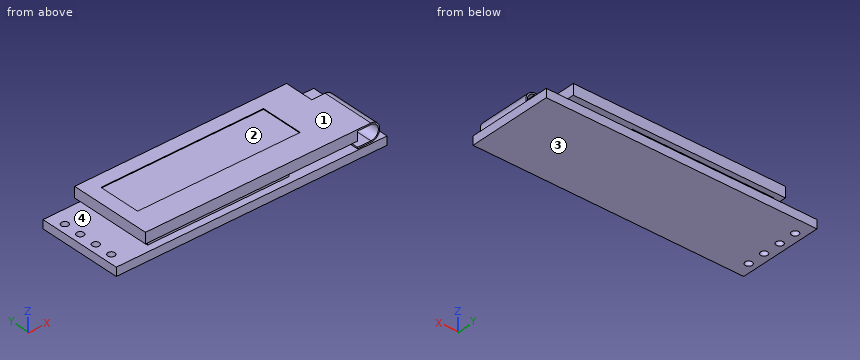
```python
from build123d import *

# Parameters (mm, degrees)
SKETCH_W     = 38.3
SKETCH_H     = 12
SKETCH_R     = 0.5
PAD_DEPTH    = 1.2
SKETCH001_W  = 20
SKETCH001_H  = 10
PAD001_DEPTH = 1
SKETCH002_W  = 30
SKETCH002_H  = 11.6
PAD002_DEPTH = 1.5
PAD003_DEPTH = 7.5
SKETCH004_W  = 23
SKETCH004_H  = 6
POCKET_DEPTH = 0.1


with BuildPart() as part:
    # Sketch → Pad (new body)
    with BuildSketch(Plane.XY):
        with Locations((17.95, 3.8)):
            Rectangle(SKETCH_W, SKETCH_H)
        Circle(SKETCH_R, mode=Mode.SUBTRACT)
        with Locations((0, 2.54)):
            Circle(SKETCH_R, mode=Mode.SUBTRACT)
        with Locations((0, 5.08)):
            Circle(SKETCH_R, mode=Mode.SUBTRACT)
        with Locations((0, 7.62)):
            Circle(SKETCH_R, mode=Mode.SUBTRACT)
    extrude(amount=PAD_DEPTH)

    # Sketch001 (on Face10 of Pad) → Pad001 (join)
    with BuildSketch(Plane.XY.offset(1.2)):
        with Locations((14.1, 3.8)):
            Rectangle(SKETCH001_W, SKETCH001_H)
    extrude(amount=PAD001_DEPTH)

    # Sketch002 (on Face15 of Pad001) → Pad002 (join)
    with BuildSketch(Plane.XY.offset(2.2)):
        with Locations((18.1, 3.8)):
            Rectangle(SKETCH002_W, SKETCH002_H)
    extrude(amount=PAD002_DEPTH)

    # Sketch003 (on Face6 of Pad002) → Pad003 (join)
    with BuildSketch(Plane.XZ.offset(2)):
        with BuildLine():
            ThreePointArc((35, 1.2), (36.25, 2.45), (35, 3.7))
            Line((33.1, 3.7), (35, 3.7))
            Line((33.1, 3.7), (33.1, 3.5))
            Line((33.1, 3.5), (35, 3.5))
            ThreePointArc((35, 1.4), (36.05, 2.45), (35, 3.5))
            Line((33.1, 1.4), (35, 1.4))
            Line((33.1, 1.4), (33.1, 1.2))
            Line((33.1, 1.2), (35, 1.2))
        make_face()
    extrude(amount=-PAD003_DEPTH)

    # Sketch004 (on Face5 of Pad003) → Pocket (cut)
    with BuildSketch(Plane.XY.offset(3.7)):
        with Locations((16.6, 4.6)):
            Rectangle(SKETCH004_W, SKETCH004_H)
    extrude(amount=-POCKET_DEPTH, mode=Mode.SUBTRACT)


solid = part.part
```
Check sheet for the modelled part. Datum: model origin and axes. Units: mm. Face numbers are marked on the shaded views. A direction names the side the tool comes from. Round coordinates to 2 decimals unless told otherwise and drop trailing zeros. Order: outer loops, then holes, each group sorted by start corner. A loop starts at its lowest first (then second) coordinate and runs counter-clockwise, first axis right, second up. Notation, with made-up numbers: (34, -0.75) - (66, -0.75) arc R24 cw to (66, 32.25) - close; hole circle Ø1 at (71, 85.25). An arc over 180 degrees is marked (long way). Write item = value, one per line.
Q1. Tool access check on the marked faces 3 and 4. Record the directions out of +Z, -Z, +X, -X, +Y, -Y that give a thin tool (end or side, any length) a straight path to the whole face; none if there is none.
Computed:
face_3 = -Z, +X, -X, +Y, -Y
face_4 = none
Q2. Section check A-A (y = 0). Record the boundary of the cut face in (x, z), and give its area (3 significant figures).
Computed:
outline = (-1.2, 0) - (-0.5, 0) - (-0.5, 1.2) - (-1.2, 1.2) - close; (0.5, 0) - (37.1, 0) - (37.1, 1.2) - (35, 1.2) arc R1.25 ccw to (35, 3.7) - (3.1, 3.7) - (3.1, 2.2) - (4.1, 2.2) - (4.1, 1.2) - (0.5, 1.2) - close; hole (24.1, 1.2) - (33.1, 1.2) - (33.1, 1.4) - (35, 1.4) arc R1.05 ccw to (35, 3.5) - (33.1, 3.5) - (33.1, 2.2) - (24.1, 2.2) - close
area = 111 mm^2
Q3. Section check B-B (x = 17). Record the boundary of the cut face in (y, z).
Computed:
outline = (-2.2, 0) - (9.8, 0) - (9.8, 1.2) - (8.8, 1.2) - (8.8, 2.2) - (9.6, 2.2) - (9.6, 3.7) - (7.6, 3.7) - (7.6, 3.6) - (1.6, 3.6) - (1.6, 3.7) - (-2, 3.7) - (-2, 2.2) - (-1.2, 2.2) - (-1.2, 1.2) - (-2.2, 1.2) - close
Q4. Go/stop test with flat-tipped pins: pin 1 (6 mm diameter, centred on x = 13, y = 2.5, fed in from +Z); pin 2 (0.5 mm diameter, centred on x = 16.5, z = 2, fed in from -Y); pin 3 (0.8 mm diameter, centred on y = 6, z = 3, fed in from -X); pin 4 (0.5 mm diameter, centred on y = 5, z = 1.5, fed in from +X). Record where each tip stops, or that it passes through.
Computed:
pin_1 = 3.7
pin_2 = -2
pin_3 = 3.1
pin_4 = 36.04
Q5. Draft check along Y on the marked faces 1 and 2. Enter one of: pulls with the +Y half, pulls with the -Y half, needs draft (parallel to the pull), parting line crosses it, or undercut.
Computed:
face_1 = needs draft
face_2 = undercut
Q6. Section check C-C (y = 5.08). Record the boundary of the cut face in (x, z).
Computed:
outline = (-1.2, 0) - (-0.5, 0) - (-0.5, 1.2) - (-1.2, 1.2) - close; (0.5, 0) - (37.1, 0) - (37.1, 1.2) - (35, 1.2) arc R1.25 ccw to (35, 3.7) - (28.1, 3.7) - (28.1, 3.6) - (5.1, 3.6) - (5.1, 3.7) - (3.1, 3.7) - (3.1, 2.2) - (4.1, 2.2) - (4.1, 1.2) - (0.5, 1.2) - close; hole (24.1, 1.2) - (33.1, 1.2) - (33.1, 1.4) - (35, 1.4) arc R1.05 ccw to (35, 3.5) - (33.1, 3.5) - (33.1, 2.2) - (24.1, 2.2) - close
Q7. Thickness scan on line 1 along Y through (x, z) = (0, 0.95); line 2 along Z through (x, y) = (33.5, 3); line 3 along Z through (x, y) = (33, 2.25). Record the ranges inside material, lowest first.
Computed:
line_1 = -2.2 to -0.5, 0.5 to 2.04, 3.04 to 4.58, 5.58 to 7.12, 8.12 to 9.8
line_2 = 0 to 1.4, 3.5 to 3.7
line_3 = 0 to 1.2, 2.2 to 3.7
